from build123d import *

# Parameters (mm, degrees)
CROQUIS1_W              = 40
CROQUIS1_H              = 28
CROQUIS1_W_2            = 3
CROQUIS1_H_2            = 15.5
SALIENTE_EXTRUIR1_DEPTH = 2.5
CROQUIS2_W              = 20
CROQUIS2_H              = 20
SALIENTE_EXTRUIR2_DEPTH = 3
SALIENTE_EXTRUIR3_DEPTH = 17.5
CROQUIS4_W              = 20
CROQUIS4_H              = 15
SALIENTE_EXTRUIR4_DEPTH = 2


with BuildPart() as part:
    # Croquis1 → Saliente-Extruir1 (new, symmetric)
    with BuildSketch(Plane.XY):
        Rectangle(CROQUIS1_W, CROQUIS1_H)
        with Locations((14.8, 0)):
            Rectangle(CROQUIS1_W_2, CROQUIS1_H_2, mode=Mode.SUBTRACT)
        with Locations((-14.8, 0)):
            Rectangle(CROQUIS1_W_2, CROQUIS1_H_2, mode=Mode.SUBTRACT)
    extrude(amount=SALIENTE_EXTRUIR1_DEPTH, both=True)

    # Croquis2 → Saliente-Extruir2 (add)
    with BuildSketch(Plane.XY.offset(2.5)):
        Rectangle(CROQUIS2_W, CROQUIS2_H)
    extrude(amount=SALIENTE_EXTRUIR2_DEPTH)

    # Croquis3 → Saliente-Extruir3 (add, symmetric)
    with BuildSketch(Plane(origin=(0, 0, 0), x_dir=(0, 0, -1), z_dir=(1, 0, 0))):
        Polygon((-2.5, -14), (-20.17766953, 3.67766953), (-15.17766953, 3.67766953), (-2.5, -9), align=None)
    extrude(amount=SALIENTE_EXTRUIR3_DEPTH, both=True)

    # Croquis4 → Saliente-Extruir4 (add)
    with BuildSketch(Plane(origin=(0, -8.25, 8.25), x_dir=(1, 0, 0), z_dir=(0, -0.7071067811865441, 0.707106781186551))):
        with Locations((0, 2.5)):
            Rectangle(CROQUIS4_W, CROQUIS4_H)
    extrude(amount=SALIENTE_EXTRUIR4_DEPTH)


solid = part.part
Read the model definition and answer for the solid it produces. Units are mm, in the model's axes. A direction names the side the tool comes from. Coordinates: 2 decimals unless noted, no trailing zeros. Order: outer loops, then holes, each group sorted by start corner. A loop starts at its lowest first (then second) coordinate and runs counter-clockwise, first axis right, second up. Notation, with made-up numbers: (88.5, -3) -> (117.5, -3) arc R13 ccw to (117.5, 9) -> close; hole circle Ø4 at (65.25, -5). An arc over 180 degrees is marked (long way). Answer as a JSON object with one key per item and string values.
1) A cutting plane is placed at B-B, the plane x = 14. Determine the outline of the cut face in (y, z).
Model answer:
{"outline": "(-14, -2.5) -> (-7.75, -2.5) -> (-7.75, 2.5) -> (-9, 2.5) -> (3.68, 15.18) -> (3.68, 20.18) -> (-14, 2.5) -> close; (7.75, -2.5) -> (14, -2.5) -> (14, 2.5) -> (7.75, 2.5) -> close"}
2) A tool of negligible diameter and unlimited length cuts with its end or side. For faces 4 (the face through (-15, -7.75, 0)), 5 (the face through (-15, 7.75, 0)), 6 (the face through (-10, -7, 11)), from which of +Z, -Z, +X, -X, +Y, -Y can it reach the whole face along a straight path? Write none if from no direction.
Model answer:
{"face 4": "-Z", "face 5": "+Z, -Z", "face 6": "+Z, -X, -Y"}
3) A cutting plane is placed at A-A, the plane y = 5.5. Determine the outline of the cut face in (x, z), plus the area to 3 significant figures.
Model answer:
{"outline": "(-20, -2.5) -> (-16.3, -2.5) -> (-16.3, 2.5) -> (-20, 2.5) -> close; (-13.3, -2.5) -> (13.3, -2.5) -> (13.3, 2.5) -> (10, 2.5) -> (10, 5.5) -> (-10, 5.5) -> (-10, 2.5) -> (-13.3, 2.5) -> close; (16.3, -2.5) -> (20, -2.5) -> (20, 2.5) -> (16.3, 2.5) -> close", "area": "230 mm²"}
4) The mould has two halves that part along Y. Classify faces 1 (the face through (-17.5, -4, 10)), 2 (the face through (-0.14, -1.88, 16.02)), 3 (the face through (0, 14, 0)): released by +Y, released by -Y, zero draft, split by the parting line, or undercut.
Model answer:
{"face 1": "zero draft", "face 2": "undercut", "face 3": "released by +Y"}
5) A cutting plane is placed at C-C, the plane y = 0.75. Determine the outline of the cut face in (x, z).
Model answer:
{"outline": "(-20, -2.5) -> (-16.3, -2.5) -> (-16.3, 2.5) -> (-20, 2.5) -> close; (-17.5, 12.25) -> (17.5, 12.25) -> (17.5, 17.25) -> (-17.5, 17.25) -> close; (-13.3, -2.5) -> (13.3, -2.5) -> (13.3, 2.5) -> (10, 2.5) -> (10, 5.5) -> (-10, 5.5) -> (-10, 2.5) -> (-13.3, 2.5) -> close; (16.3, -2.5) -> (20, -2.5) -> (20, 2.5) -> (16.3, 2.5) -> close"}
6) Each of these flat-tipped pins is pushed along its axis until it touches: pin 1 (10 mm diameter, centred on y = -8, z = 16, fed in from +X); pin 2 (9 mm diameter, centred on y = -9, z = 9, fed in from -X); pin 3 (1.5 mm diameter, centred on x = -12, z = 4.5, fed in from -Y); pin 4 (2 mm diameter, centred on y = -11, z = 10, fed in from +X). Where does it stop, or does it pass through?
Model answer:
{"pin 1": "stops at x = 10", "pin 2": "stops at x = -17.5", "pin 3": "stops at y = -12.75", "pin 4": "passes through"}
7) Consider line 1 along Y through (x, z) = (-13.5, 0); line 2 along X through (y, z) = (0.5, -1.5); line 3 along Y through (x, z) = (13.5, 14). Determine where each line is inside the solid, lowest interval first. Write a range as from..to.
Model answer:
{"line 1": "y = -14..-7.75, 7.75..14", "line 2": "x = -20..-16.3, -13.3..13.3, 16.3..20", "line 3": "y = -2.5..2.5"}
8) A cutting plane is placed at D-D, the plane x = -2. Determine the outline of the cut face in (y, z), plus the area to 3 significant figures.
Model answer:
{"outline": "(-14, -2.5) -> (14, -2.5) -> (14, 2.5) -> (10, 2.5) -> (10, 5.5) -> (-6, 5.5) -> (3.68, 15.18) -> (3.68, 20.18) -> (-1.18, 15.32) -> (-2.59, 16.74) -> (-13.2, 6.13) -> (-11.79, 4.71) -> (-14, 2.5) -> close", "area": "298 mm²"}
